Could you check a few things on this drawing? It's one solid part, dimensions in mm from its lowest x, y, z. A direction names the side the tool comes from. Coordinates: 2 decimals unless noted, no trailing zeros. Order: outer loops, then holes, each group sorted by start corner. A loop starts at its lowest first (then second) coordinate and runs counter-clockwise, first axis right, second up. Notation, with made-up numbers: M 75.5,36.25 L 111.5,36.25 A5 cw 111.5,45.25 Z; hole C 38,2 d7. An arc over 180 degrees is marked long. One line per question, with ' | ' between items. Start each with the question number.
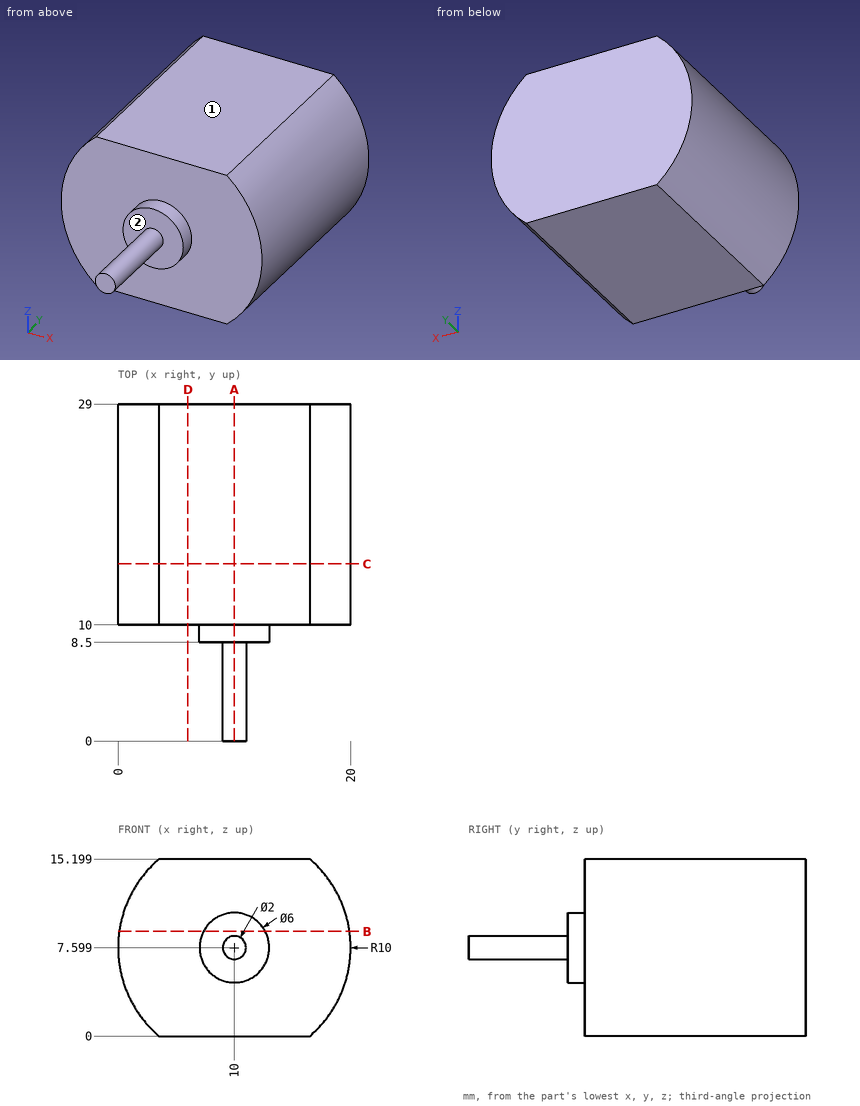
1. Imagine slicing it at B-B (z = 9). List the corners of the cut face in (x, y) for me, then the cut area to 3 significant figures.
2. Which directions (+Z, -Z, +X, -X, +Y, -Y) give clear straight access to the entire face, cutting with the end or side of a thin tool? Please do the marked faces 1 and 2.
3. Imagine slicing it at D-D (x = 6). List the corners of the cut face in (y, z) for me, then the cut area to 3 significant figures.
4. Imagine slicing it at C-C (y = 15.25). List the corners of the cut face in (x, z) for me, then the cut area to 3 significant figures.
5. Will these pins go through, and if not, where does the flat tip stop? pin 1 (8 mm diameter, centred on x = 17.5, y = 7, fed in from +Z); pin 2 (1.5 mm diameter, centred on y = 19, z = 13, fed in from -X); pin 3 (8 mm diameter, centred on y = 5, z = 9, fed in from -X).
6. Imagine slicing it at A-A (x = 10). List the corners of the cut face in (y, z) for me.
7. I need wall thicknesses on line 1 (Y direction, x = 13.25, z = 13.75); line 2 (X direction, y = 20, z = 7.5); line 3 (Y direction, x = 11.5, z = 6). Which ranges of each line are inside material? Lowest first, please.
Entries:
1) outline: M 0.1,10 L 7.35,10 L 7.35,8.5 L 12.65,8.5 L 12.65,10 L 19.9,10 L 19.9,29 L 0.1,29 Z | area: 384 mm²
2) face 1: +Z, +X, -X, +Y, -Y | face 2: -Y
3) outline: M 10,0 L 29,0 L 29,15.2 L 10,15.2 Z | area: 289 mm²
4) outline: M 3.5,0 L 16.5,0 A10 ccw 16.5,15.2 L 3.5,15.2 A10 ccw Z | area: 271 mm²
5) pin 1: z = 15.2 | pin 2: x = 1.15 | pin 3: x = 7
6) outline: M 0,6.6 L 8.5,6.6 L 8.5,4.6 L 10,4.6 L 10,0 L 29,0 L 29,15.2 L 10,15.2 L 10,10.6 L 8.5,10.6 L 8.5,8.6 L 0,8.6 Z
7) line 1: 10 to 29 | line 2: 0 to 20 | line 3: 8.5 to 29
